from build123d import *

# Parameters (mm, degrees)
F0_W     = 76.2
F0_H     = 76.2
F1_DEPTH = 69.85
F2_T     = -25.4
F3_T     = -2.54


with BuildPart() as f1:
    # F0 (on Right) → F1 (new body)
    with BuildSketch(Plane.YZ):
        Rectangle(F0_W, F0_H)
    extrude(amount=F1_DEPTH)

    # F2
    f2_openings = [f1.faces().sort_by_distance(p)[0] for p in [
        (0, 0, 0),
    ]]
    offset(amount=F2_T, openings=f2_openings)

    # F3
    f3_openings = [f1.faces().sort_by_distance(p)[0] for p in [
        (69.85, 0, 0),
    ]]
    offset(amount=F3_T, openings=f3_openings, kind=Kind.INTERSECTION)


solid = f1.part
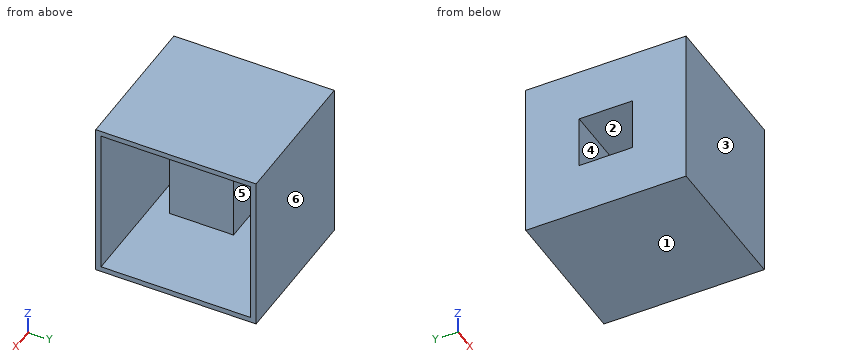
CAD build for the part. Positions are in the model's coordinates, mm. Face numbers are marked on the shaded views. A direction names the side the tool comes from. Give positions to 0.01 mm unless a question says otherwise; leave off trailing zeros. Write each loop counter-clockwise with the first axis right and the second up, starting at its lowest first coordinate (ties: lowest second). Pieces come first, ordered by that corner, then holes. Notation, with made-up numbers: (29, -27.75) - (73, -27.75) arc R27 cw to (73, 9.25) - close; hole circle Ø3 at (10, 20.5). An arc over 180 degrees is marked (long way). Put each result on its own line as item: value.
(1) Saw through at A-A (x = 40). List the corners of the cut face in (y, z).
Working result:
outline: (-38.1, -38.1) - (38.1, -38.1) - (38.1, 38.1) - (-38.1, 38.1) - close; (-15.24, -15.24) - (15.24, -15.24) - (15.24, 15.24) - (-15.24, 15.24) - close; hole (-35.56, -35.56) - (35.56, -35.56) - (35.56, 35.56) - (-35.56, 35.56) - close; hole (-12.7, -12.7) - (12.7, -12.7) - (12.7, 12.7) - (-12.7, 12.7) - close
(2) Wall check: L1, parallel to Y at x = 23.5, z = -5.5; L2, parallel to Y at x = 28, z = -13. Give the ranges that are in metal, low to high.
Working result:
L1: -38.1 to -35.56, -15.24 to -12.7, 12.7 to 15.24, 35.56 to 38.1
L2: -38.1 to -35.56, -15.24 to 15.24, 35.56 to 38.1
(3) Tool access for the marked faces 4, 5 and 6: list every direction of +Z, -Z, +X, -X, +Y, -Y with a clear straight run to the whole face (end or side of a thin tool).
Working result:
face 4: -X
face 5: +X
face 6: +Z, -Z, +X, -X, +Y
(4) Pull direction Z, two halves, no side cores. Call the marked faces 1, 2 and 3: released by +Z, released by -Z, zero draft, split by the parting line, or undercut.
Working result:
face 1: released by -Z
face 2: undercut
face 3: zero draft
(5) Saw through at D-D (x = 49). List the corners of the cut face in (y, z).
Working result:
outline: (-38.1, -38.1) - (38.1, -38.1) - (38.1, 38.1) - (-38.1, 38.1) - close; hole (-35.56, -35.56) - (35.56, -35.56) - (35.56, 35.56) - (-35.56, 35.56) - close
(6) Saw through at B-B (z = -28.5). List the corners of the cut face in (x, y).
Working result:
outline: (0, -38.1) - (69.85, -38.1) - (69.85, -35.56) - (2.54, -35.56) - (2.54, 35.56) - (69.85, 35.56) - (69.85, 38.1) - (0, 38.1) - close
(7) Saw through at C-C (y = 4). List the corners of the cut face in (x, z), then the cut area to 3 significant figures.
Working result:
outline: (0, -38.1) - (69.85, -38.1) - (69.85, -35.56) - (2.54, -35.56) - (2.54, -15.24) - (46.99, -15.24) - (46.99, 15.24) - (2.54, 15.24) - (2.54, 35.56) - (69.85, 35.56) - (69.85, 38.1) - (0, 38.1) - (0, 12.7) - (44.45, 12.7) - (44.45, -12.7) - (0, -12.7) - close
area: 761 mm^2
(8) Drop flat-ended pins along their axis: pin 1 Ø2 at (y, z) = (-8.5, -8) entering from +X; pin 2 Ø12.5 at (y, z) = (0, -2) entering from -X. Give the stop position or say it passes through.
Working result:
pin 1: x = 46.99
pin 2: x = 44.45
